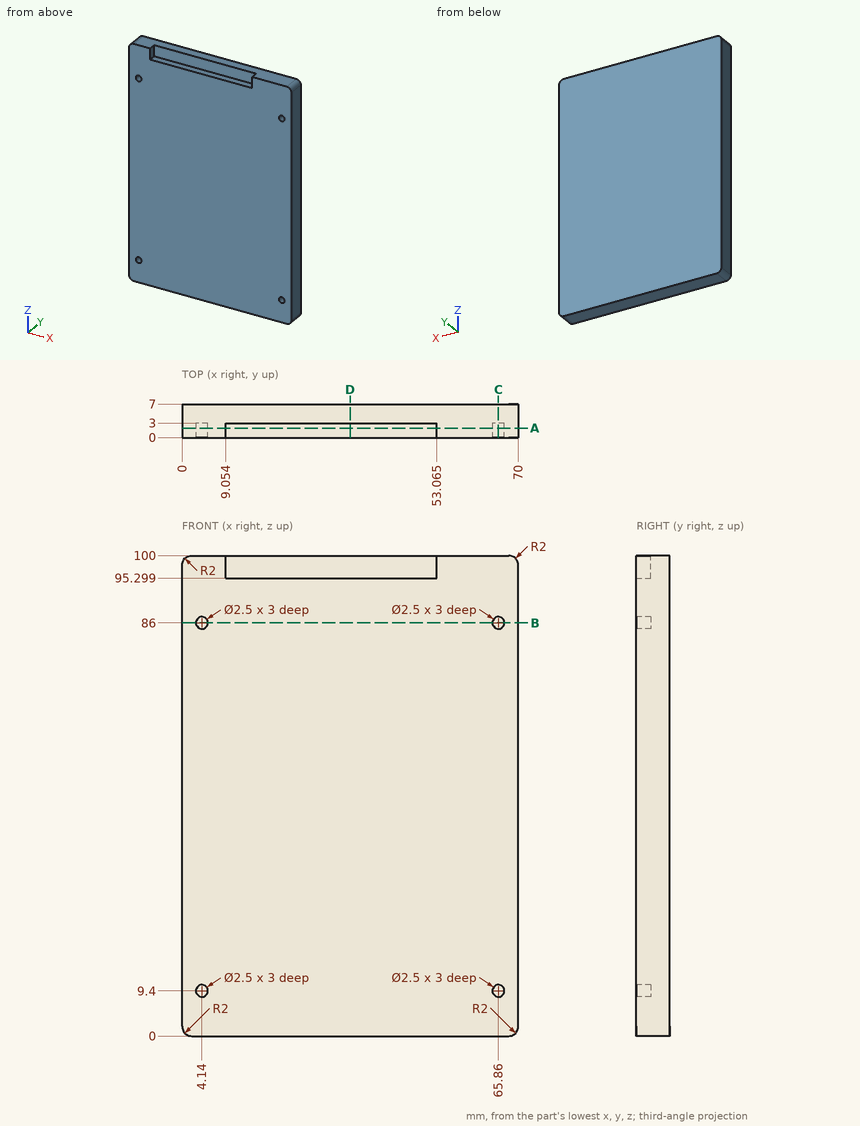
Source: three-view drawing plus pictorial views. Frame: mm from the lowest corner of the part. Give positions to 0.01 mm unless a question says otherwise; leave off trailing zeros. Order: outer loops, then holes, each group sorted by start corner. A loop starts at its lowest first (then second) coordinate and runs counter-clockwise, first axis right, second up. Notation, with made-up numbers: (34, 68) - (48, 68) arc R28 ccw to (48, 91) - close; hole circle Ø6 at (-33.75, 71.25). An arc over 180 degrees is marked (long way). Answer as a JSON object with one key per item and string values. Group by question number.
Q1. Cut plane D-D, the plane x = 35. Output: boundary loops of the cut face in (y, z), then the cut area to 3 significant figures.
Q2. Line query: probe 1 along Z at (x, y) = (65.86, 1.95); probe 2 along X at (y, z) = (2.4, 86); probe 3 along Z at (x, y) = (20, 1). Output: solid intervals per line, ascending.
Q3. First-contact query: pin 1 Ø3.5 at (x, y) = (30.5, 1.5) entering from +Z; pin 2 Ø2 at (x, z) = (4, 86) entering from -Y. Flat tips, straight axial feed; report the tip coordinate or a pass-through.
Q4. Cut plane A-A, the plane y = 2. Count the separate pieces of the cut face and the enclosed holes in it, then the cut area to 3 significant figures.
Q5. Cut plane B-B, the plane z = 86. Output: boundary loops of the cut face in (x, y).
Q6. Cut plane C-C, the plane x = 65.86. Output: boundary loops of the cut face in (y, z), then the cut area to 3 significant figures.
Results:
{
 "1": {"outline": "(0, 0) - (7, 0) - (7, 100) - (3, 100) - (3, 95.3) - (0, 95.3) - close", "area": "686 mm^2"},
 "2": {"probe 1": "0 to 8.15, 10.65 to 84.75, 87.25 to 100", "probe 2": "0 to 2.89, 5.39 to 64.61, 67.11 to 70", "probe 3": "0 to 95.3"},
 "3": {"pin 1": "z = 100", "pin 2": "y = 3"},
 "4": {"separate pieces": "1", "enclosed holes": "4", "area": "6,770 mm^2"},
 "5": {"outline": "(0, 0) - (2.89, 0) - (2.89, 3) - (5.39, 3) - (5.39, 0) - (64.61, 0) - (64.61, 3) - (67.11, 3) - (67.11, 0) - (70, 0) - (70, 7) - (0, 7) - close"},
 "6": {"outline": "(0, 0) - (7, 0) - (7, 100) - (0, 100) - (0, 87.25) - (3, 87.25) - (3, 84.75) - (0, 84.75) - (0, 10.65) - (3, 10.65) - (3, 8.15) - (0, 8.15) - close", "area": "685 mm^2"}
}
